Check sheet for the drawn part. Datum: minimum x, y, z corner. Units: mm. A direction names the side the tool comes from. Coordinates: 2 decimals unless noted, no trailing zeros. Write each loop counter-clockwise with the first axis right and the second up, starting at its lowest first coordinate (ties: lowest second). Pieces come first, ordered by that corner, then holes. Notation, with made-up numbers: M -39.5,13 L 14.5,13 A20 ccw 14.5,17 Z; hole C -21,60 d6. An arc over 180 degrees is marked long. Write item = value, one per line. Start each with the question number.
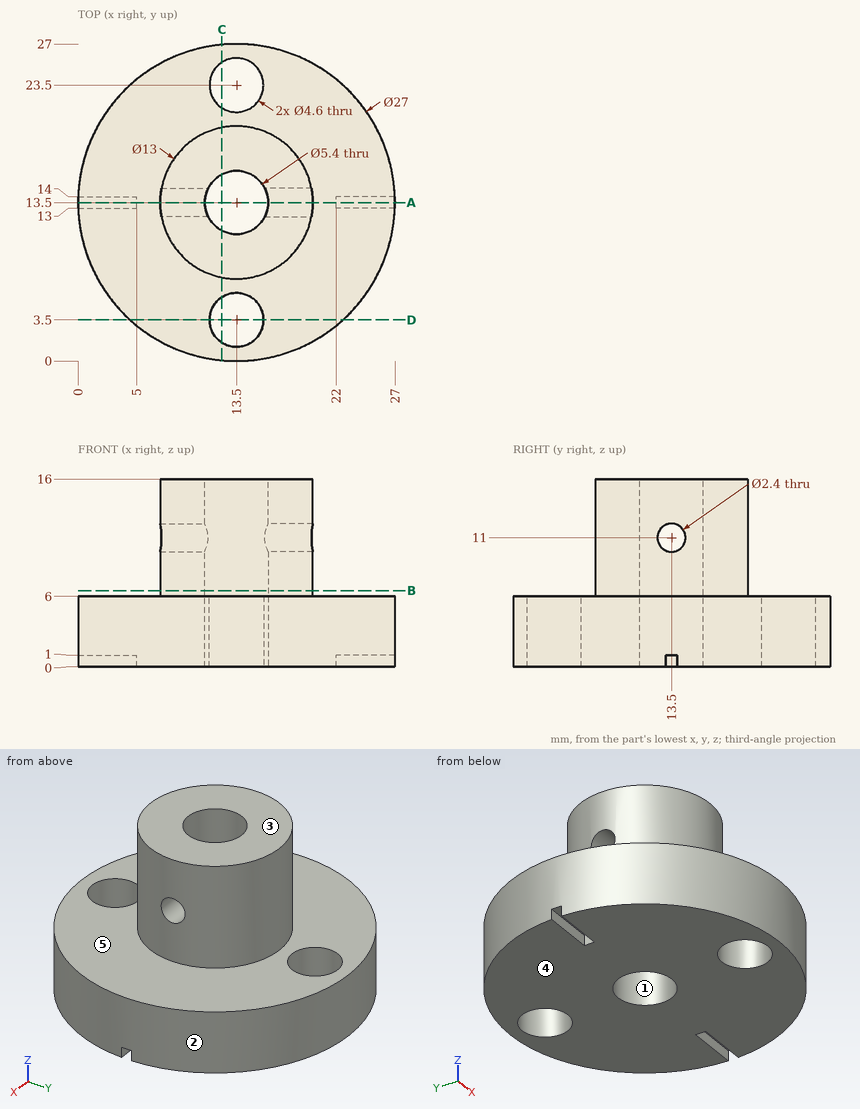
Q1. Set-up check for the marked faces 4 and 5: record each of +Z, -Z, +X, -X, +Y, -Y from which the full face is reachable in a straight line by a thin tool's end or side.
Q2. Scan lines: L1, parallel to Y at x = 13.5, z = 3.75; L2, parallel to X at y = 13.5, z = 6.5; L3, parallel to Y at x = 15.5, z = 1.25. Record each from-to range of solid material in increasing order.
Q3. Gauge pin test, flat ends, axial feed: pin 1 (3 mm diameter, centred on y = 13.5, z = 11, fed in from +X); pin 2 (0.5 mm diameter, centred on y = 13.5, z = 0.5, fed in from -X); pin 3 (1.5 mm diameter, centred on x = 16.5, z = 7, fed in from +Y); pin 4 (2 mm diameter, centred on y = 13.5, z = 11, fed in from +X). Record the tip position at first contact, or that the pin passes through.
Q4. Draft check along Y on the marked faces 1, 2 and 3. Enter one of: pulls with the +Y half, pulls with the -Y half, needs draft (parallel to the pull), parting line crosses it, or undercut.
Q5. Cross-section at A-A on y = 13.5. Enter the section's corners in (x, z), and give its area (3 significant figures).
Q6. Cross-section at C-C on x = 12.25. Enter the section's corners in (y, z).
Q7. Cross-section at D-D on y = 3.5. Enter the section's corners in (x, z).
Q8. Cross-section at B-B on z = 6.5. Enter the section's corners in (x, y), and give its area (3 significant figures).
Values found:
q1.face_4 = -Z, +X, -X, +Y, -Y
q1.face_5 = +Z
q2.L1 = 0 to 1.2, 5.8 to 10.8, 16.2 to 21.2, 25.8 to 27
q2.L2 = 7 to 10.8, 16.2 to 20
q2.L3 = 0.15 to 2.36, 4.64 to 11.69, 15.31 to 22.36, 24.64 to 26.85
q3.pin_1 = 20
q3.pin_2 = 5
q3.pin_3 = 19.6
q3.pin_4 = through
q4.face_1 = undercut
q4.face_2 = parting line crosses it
q4.face_3 = needs draft
q5.outline = M 0,1 L 5,1 L 5,0 L 10.8,0 L 10.8,9.8 L 7,9.8 L 7,6 L 0,6 Z; M 7,12.2 L 10.8,12.2 L 10.8,16 L 7,16 Z; M 16.2,0 L 22,0 L 22,1 L 27,1 L 27,6 L 20,6 L 20,9.8 L 16.2,9.8 Z; M 16.2,12.2 L 20,12.2 L 20,16 L 16.2,16 Z
q5.area = 177 mm²
q6.outline = M 0.06,0 L 1.57,0 L 1.57,6 L 0.06,6 Z; M 5.43,0 L 11.11,0 L 11.11,16 L 7.12,16 L 7.12,6 L 5.43,6 Z; M 15.89,0 L 21.57,0 L 21.57,6 L 19.88,6 L 19.88,16 L 15.89,16 Z; M 25.43,0 L 26.94,0 L 26.94,6 L 25.43,6 Z
q7.outline = M 4.43,0 L 11.2,0 L 11.2,6 L 4.43,6 Z; M 15.8,0 L 22.57,0 L 22.57,6 L 15.8,6 Z
q8.outline = C 13.5,13.5 d13; hole C 13.5,13.5 d5.4
q8.area = 110 mm²
